Geometry check sheet. Reference: the model listing, model coordinates, mm. A direction names the side the tool comes from. Give positions to 0.01 mm unless a question says otherwise; leave off trailing zeros. Loops run counter-clockwise (first coordinate to the right, second up) from the corner with the lowest first, then second, coordinate; pieces in that order, holes last. Notation, with made-up numbers: (52.5, -22.5) -> (102.5, -22.5) arc R17 ccw to (102.5, -6.5) -> close; hole circle Ø7 at (-3, -24). An arc over 180 degrees is marked (long way). Answer as a JSON object with one key per item and string values.
from build123d import *

# Parameters (mm, degrees)
BOSS_EXTRU_1_DEPTH           = 20
ENL_V_MAT_EXTRU_1_DEPTH      = 34
ENL_V_MAT_EXTRU_2_DEPTH      = 140.70683591
ENL_V_MAT_EXTRU_2_DEPTH_BACK = 2
ESQUISSE3_R                  = 11
ESQUISSE3_R_2                = 16


with BuildPart() as part:
    # Esquisse1 → Boss.-Extru.1 (new, symmetric)
    with BuildSketch(Plane.XY):
        with BuildLine():
            Line((0, 21), (60, 61))
            ThreePointArc((60, 61), (121, 0), (60, -61))
            Line((60, -61), (0, -21))
            ThreePointArc((0, -21), (-21, 0), (0, 21))
        make_face()
    extrude(amount=BOSS_EXTRU_1_DEPTH, both=True)

    # Esquisse2 → Enlèv. mat.-Extru.1 (cut)
    with BuildSketch(Plane.XY.offset(20)):
        with BuildLine():
            Line((0, 17), (60, 57))
            ThreePointArc((60, 57), (117, 0), (60, -57))
            Line((60, -57), (0, -17))
            ThreePointArc((0, -17), (-17, 0), (0, 17))
        make_face()
    extrude(amount=-ENL_V_MAT_EXTRU_1_DEPTH, mode=Mode.SUBTRACT)

    # Esquisse3 → Enlèv. mat.-Extru.2 (cut, two sides: drawn at the far end of the back side and taken through both)
    with BuildSketch(Plane.XY.offset(-14).offset(-ENL_V_MAT_EXTRU_2_DEPTH_BACK)):
        Circle(ESQUISSE3_R)
        with Locations((60, 0)):
            Circle(ESQUISSE3_R_2)
    extrude(amount=ENL_V_MAT_EXTRU_2_DEPTH + ENL_V_MAT_EXTRU_2_DEPTH_BACK, mode=Mode.SUBTRACT)


solid = part.part
1) Section check D-D on y = 4. Record the cut outline in (x, z), plus the area to 3 significant figures.
Geometry check:
{"outline": "(-20.62, -20) -> (120.87, -20) -> (120.87, 20) -> (116.86, 20) -> (116.86, -14) -> (75.49, -14) -> (75.49, -16) -> (44.51, -16) -> (44.51, -14) -> (10.25, -14) -> (10.25, -16) -> (-10.25, -16) -> (-10.25, -14) -> (-16.52, -14) -> (-16.52, 20) -> (-20.62, 20) -> close", "area": "1,020 mm2"}
2) Section check C-C on y = 23.5. Record the cut outline in (x, z), plus the area to 3 significant figures.
Geometry check:
{"outline": "(3.75, -20) -> (116.29, -20) -> (116.29, 20) -> (111.93, 20) -> (111.93, -14) -> (9.75, -14) -> (9.75, 20) -> (3.75, 20) -> close", "area": "1,030 mm2"}
3) Section check A-A on z = 8.5. Record the cut outline in (x, y), plus the area to 3 significant figures.
Geometry check:
{"outline": "(0, -21) -> (60, -61) arc R61 ccw to (60, 61) -> (0, 21) arc R21 ccw to start; hole (0, -17) -> (60, -57) arc R57 ccw to (60, 57) -> (0, 17) arc R17 ccw to start", "area": "1,460 mm2"}
4) Section check B-B on x = 22.5. Record the cut outline in (y, z), plus the area to 3 significant figures.
Geometry check:
{"outline": "(-36, -20) -> (36, -20) -> (36, 20) -> (32, 20) -> (32, -14) -> (-32, -14) -> (-32, 20) -> (-36, 20) -> close", "area": "704 mm2"}
5) Tool access check on faces 1 (the face through (116.986, 1.253, 3.238)), 2 (the face through (30, -41, 0)). Record the directions out of +Z, -Z, +X, -X, +Y, -Y that give a thin tool (end or side, any length) a straight path to the whole face; none if there is none.
Geometry check:
{"face 1": "+Z", "face 2": "+Z, -Z, -X, -Y"}
6) Draft check along X on faces 3 (the face through (34.6, -40.4, 20)), 4 (the face through (30, 41, 0)), 5 (the face through (-17, 0, 3)). Enter one of: pulls with the +X half, pulls with the -X half, needs draft (parallel to the pull), parting line crosses it, or undercut.
Geometry check:
{"face 3": "needs draft", "face 4": "pulls with the -X half", "face 5": "undercut"}
7) Material ranges on line 1 along X through (y, z) = (0, -15.1); line 2 along Y through (x, z) = (60, -15.2); line 3 along Z through (x, y) = (73.5, 12), recorded low to high. Write a range as from..to.
Geometry check:
{"line 1": "x = -21..-11, 11..44, 76..121", "line 2": "y = -61..-16, 16..61", "line 3": "z = -20..-14"}
8) Depth check by flat-ended pin: P1, Ø2, axis at y = -32.5, z = -14.5, coming from the -X side; P2, Ø10, axis at y = -29.5, z = -2.5, coming from the -X side; P3, Ø16, axis at x = 61, y = 0.5, coming from the +Z side. Enter the tip coordinate at first touch or a pass-through.
Geometry check:
{"P1": "stops at x = 15.75", "P2": "stops at x = 5.25", "P3": "stops at z = -16"}
